Verification items for the finished model (mm, model axes). Face numbers are marked on the shaded views. Round coordinates to 2 decimals unless told otherwise and drop trailing zeros. Order: outer loops, then holes, each group sorted by start corner. A loop starts at its lowest first (then second) coordinate and runs counter-clockwise, first axis right, second up. Notation, with made-up numbers: M 55,34.5 L 72,34.5 A15 cw 72,40.5 Z; hole C 66.25,-29 d5. An arc over 180 degrees is marked long. Answer as a JSON object with one key per item and string values. Group by question number.
```python
from build123d import *

# Parameters (mm, degrees)
BOSS_EXTRUDE1_DEPTH     = 52
SHELL1_START            = 3
SHELL1_DEPTH            = 46
SKETCH2_R               = 4.5
BOSS_EXTRUDE2_DEPTH     = 52
SKETCH3_R               = 3.25
CUT_EXTRUDE1_DEPTH      = 49
SKETCH4_R               = 1.7
CUT_EXTRUDE2_DEPTH      = 91.166512631
CUT_EXTRUDE3_DEPTH      = 20
CUT_EXTRUDE3_DEPTH_BACK = 20
CUT_EXTRUDE4_DEPTH      = 3.5
SKETCH7_R               = 4
CUT_EXTRUDE5_DEPTH      = 3.5
SKETCH8_W               = 6
SKETCH8_H               = 20
BOSS_EXTRUDE3_DEPTH     = 8
SKETCH9_W               = 1.9
SKETCH9_H               = 16.6
CUT_EXTRUDE6_DEPTH      = 6
SKETCH10_R              = 5
CUT_EXTRUDE7_DEPTH      = 3.5


# Read off the part's stored shape, not the designer's step: Shell1
with BuildPart() as part:
    # Sketch1 → Boss-Extrude1 (new body)
    with BuildSketch(Plane.XY):
        with BuildLine():
            Line((-45, -55), (45, -55))
            ThreePointArc((45, -55), (52.071067812, -52.071067812), (55, -45))
            Line((55, -45), (55, -10))
            ThreePointArc((55, -10), (52.071067812, -2.928932188), (45, 0))
            Line((45, 0), (-45, 0))
            ThreePointArc((-45, 0), (-52.071067812, -2.928932188), (-55, -10))
            Line((-55, -10), (-55, -45))
            ThreePointArc((-55, -45), (-52.071067812, -52.071067812), (-45, -55))
        make_face()
    extrude(amount=BOSS_EXTRUDE1_DEPTH)

    # Shell1 outline → Shell1 (cut)
    with BuildSketch(Plane.XY.offset(SHELL1_START)):
        with BuildLine():
            Line((45, -3), (45, 0))
            Line((45, 0), (-45, 0))
            Line((-45, 0), (-45, -3))
            ThreePointArc((-45, -3), (-49.949747468, -5.050252532), (-52, -10))
            Line((-52, -10), (-52, -45))
            ThreePointArc((-52, -45), (-49.949747468, -49.949747468), (-45, -52))
            Line((-45, -52), (45, -52))
            ThreePointArc((45, -52), (49.949747468, -49.949747468), (52, -45))
            Line((52, -45), (52, -10))
            ThreePointArc((52, -10), (49.949747468, -5.050252532), (45, -3))
        make_face()
    extrude(amount=SHELL1_DEPTH, mode=Mode.SUBTRACT)

    # Sketch2 → Boss-Extrude2 (add)
    with BuildSketch(Plane(origin=(0, 0, 0), x_dir=(1, 0, 0), z_dir=(0, 1, 0))):
        with Locations(Location((-40, -8, 0), (0, 0, 270))):
            Circle(SKETCH2_R)
        with Locations(Location((40, -8, 0), (0, 0, 270))):
            Circle(SKETCH2_R)
        with Locations(Location((-40, -40, 0), (0, 0, 270))):
            Circle(SKETCH2_R)
        with Locations(Location((40, -40, 0), (0, 0, 270))):
            Circle(SKETCH2_R)
    extrude(amount=-BOSS_EXTRUDE2_DEPTH)

    # Sketch3 → Cut-Extrude1 (cut)
    with BuildSketch(Plane.XZ.offset(55)):
        with Locations(Location((-40, 8, 0), (0, 0, 270))):
            Circle(SKETCH3_R)
        with Locations(Location((40, 8, 0), (0, 0, 270))):
            Circle(SKETCH3_R)
        with Locations(Location((-40, 40, 0), (0, 0, 270))):
            Circle(SKETCH3_R)
        with Locations(Location((40, 40, 0), (0, 0, 270))):
            Circle(SKETCH3_R)
    extrude(amount=-CUT_EXTRUDE1_DEPTH, mode=Mode.SUBTRACT)

    # Sketch4 → Cut-Extrude2 (cut, through all)
    with BuildSketch(Plane.XZ.offset(6)):
        with Locations(Location((-40, 8, 0), (0, 0, 270))):
            Circle(SKETCH4_R)
        with Locations(Location((40, 8, 0), (0, 0, 270))):
            Circle(SKETCH4_R)
        with Locations(Location((-40, 40, 0), (0, 0, 270))):
            Circle(SKETCH4_R)
        with Locations(Location((40, 40, 0), (0, 0, 270))):
            Circle(SKETCH4_R)
    extrude(amount=-CUT_EXTRUDE2_DEPTH, mode=Mode.SUBTRACT)

    # Sketch5 → Cut-Extrude3 (cut, two sides: drawn at the far end of the back side and taken through both)
    with BuildSketch(Plane.XY.offset(26).offset(-CUT_EXTRUDE3_DEPTH_BACK)):
        Polygon((-51, -14), (-51, -11.5), (-55.5, -16), (-55.5, -18.5), align=None)
        Polygon((51, -14), (51, -11.5), (55.5, -16), (55.5, -18.5), align=None)
        Polygon((-51, -20), (-51, -17.5), (-55.5, -22), (-55.5, -24.5), align=None)
        Polygon((51, -20), (51, -17.5), (55.5, -22), (55.5, -24.5), align=None)
        Polygon((-51, -26), (-51, -23.5), (-55.5, -28), (-55.5, -30.5), align=None)
        Polygon((51, -26), (51, -23.5), (55.5, -28), (55.5, -30.5), align=None)
        Polygon((-51, -32), (-51, -29.5), (-55.5, -34), (-55.5, -36.5), align=None)
        Polygon((51, -32), (51, -29.5), (55.5, -34), (55.5, -36.5), align=None)
        Polygon((-51, -38), (-51, -35.5), (-55.5, -40), (-55.5, -42.5), align=None)
        Polygon((51, -38), (51, -35.5), (55.5, -40), (55.5, -42.5), align=None)
    extrude(amount=CUT_EXTRUDE3_DEPTH + CUT_EXTRUDE3_DEPTH_BACK, mode=Mode.SUBTRACT)

    # Sketch6 → Cut-Extrude4 (cut)
    with BuildSketch(Plane.XZ.offset(55)):
        with BuildLine():
            Line((-34.5, 12), (-34.5, 40))
            ThreePointArc((-34.5, 40), (-33, 41.5), (-31.5, 40))
            Line((-31.5, 40), (-31.5, 12))
            ThreePointArc((-31.5, 12), (-33, 10.5), (-34.5, 12))
        make_face()
        with BuildLine():
            Line((-28.5, 12), (-28.5, 40))
            ThreePointArc((-28.5, 40), (-27, 41.5), (-25.5, 40))
            Line((-25.5, 40), (-25.5, 12))
            ThreePointArc((-25.5, 12), (-27, 10.5), (-28.5, 12))
        make_face()
        with BuildLine():
            Line((-22.5, 12), (-22.5, 40))
            ThreePointArc((-22.5, 40), (-21, 41.5), (-19.5, 40))
            Line((-19.5, 40), (-19.5, 12))
            ThreePointArc((-19.5, 12), (-21, 10.5), (-22.5, 12))
        make_face()
        with BuildLine():
            Line((-16.5, 12), (-16.5, 40))
            ThreePointArc((-16.5, 40), (-15, 41.5), (-13.5, 40))
            Line((-13.5, 40), (-13.5, 12))
            ThreePointArc((-13.5, 12), (-15, 10.5), (-16.5, 12))
        make_face()
        with BuildLine():
            Line((-10.5, 12), (-10.5, 40))
            ThreePointArc((-10.5, 40), (-9, 41.5), (-7.5, 40))
            Line((-7.5, 40), (-7.5, 12))
            ThreePointArc((-7.5, 12), (-9, 10.5), (-10.5, 12))
        make_face()
        with BuildLine():
            Line((-4.5, 12), (-4.5, 40))
            ThreePointArc((-4.5, 40), (-3, 41.5), (-1.5, 40))
            Line((-1.5, 40), (-1.5, 12))
            ThreePointArc((-1.5, 12), (-3, 10.5), (-4.5, 12))
        make_face()
        with BuildLine():
            Line((1.5, 12), (1.5, 40))
            ThreePointArc((1.5, 40), (3, 41.5), (4.5, 40))
            Line((4.5, 40), (4.5, 12))
            ThreePointArc((4.5, 12), (3, 10.5), (1.5, 12))
        make_face()
        with BuildLine():
            Line((7.5, 12), (7.5, 40))
            ThreePointArc((7.5, 40), (9, 41.5), (10.5, 40))
            Line((10.5, 40), (10.5, 12))
            ThreePointArc((10.5, 12), (9, 10.5), (7.5, 12))
        make_face()
        with BuildLine():
            Line((31.5, 12), (31.5, 40))
            ThreePointArc((31.5, 40), (33, 41.5), (34.5, 40))
            Line((34.5, 40), (34.5, 12))
            ThreePointArc((34.5, 12), (33, 10.5), (31.5, 12))
        make_face()
    extrude(amount=-CUT_EXTRUDE4_DEPTH, mode=Mode.SUBTRACT)

    # Sketch7 → Cut-Extrude5 (cut)
    with BuildSketch(Plane(origin=(0, 0, 0), x_dir=(-1, 0, 0), z_dir=(0, 0, -1))):
        with Locations((30, -12)):
            Circle(SKETCH7_R)
        with Locations((-30, -12)):
            Circle(SKETCH7_R)
    extrude(amount=-CUT_EXTRUDE5_DEPTH, mode=Mode.SUBTRACT)

    # Sketch8 → Boss-Extrude3 (add)
    with BuildSketch(Plane(origin=(0, -52, 0), x_dir=(1, 0, 0), z_dir=(0, 1, 0))):
        with Locations((-44, -26)):
            Rectangle(SKETCH8_W, SKETCH8_H)
    extrude(amount=BOSS_EXTRUDE3_DEPTH)

    # Sketch9 → Cut-Extrude6 (cut)
    with BuildSketch(Plane(origin=(0, -44, 0), x_dir=(1, 0, 0), z_dir=(0, 1, 0))):
        with Locations((-44, -26)):
            Rectangle(SKETCH9_W, SKETCH9_H)
    extrude(amount=-CUT_EXTRUDE6_DEPTH, mode=Mode.SUBTRACT)

    # Sketch10 → Cut-Extrude7 (cut)
    with BuildSketch(Plane.XZ.offset(55)):
        with Locations(Location((20, 26, 0), (0, 0, 270))):
            Circle(SKETCH10_R)
    extrude(amount=-CUT_EXTRUDE7_DEPTH, mode=Mode.SUBTRACT)


solid = part.part
```
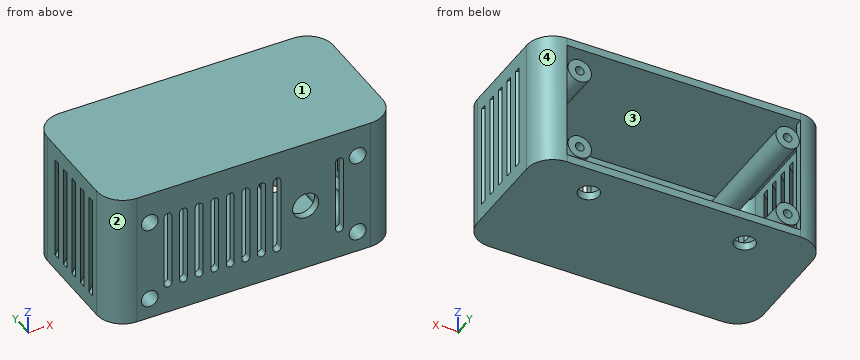
Q1. Release check for a two-part mould opening along X. For the marked faces 1, 2, 3 and 4 record: released by +X, released by -X, zero draft, split by the parting line, or undercut.
Q2. Cross-section at C-C, the plane z = 28. Give the number of separate pieces and of enclosed holes in the cut face, then the cut area to 3 significant figures.
Q3. Gauge pin test, flat ends, axial feed: pin 1 Ø3.5 at (y, z) = (-54, 29.5) entering from -X; pin 2 Ø2.5 at (y, z) = (-1, 27.5) entering from -X; pin 3 Ø6 at (x, z) = (-1, 12.5) entering from +Y. Record the tip position at first contact, or that the pin passes through.
Q4. Cross-section at B-B, the plane x = 20. Record the cut outline in (y, z), then the cut area to 3 significant figures.
Q5. Thickness scan on line 1 (Z direction, x = -4, y = -47.5); line 2 (X direction, y = -12, z = 47.5); line 3 (Z direction, x = -38.5, y = -38). Record the ranges inside material, lowest first. Write a range as from..to.
Q6. Cross-section at A-A, the plane x = -21. Record the cut outline in (y, z).
Conclusion:
{
 "1": {"face 1": "zero draft", "face 2": "released by -X", "face 3": "undercut", "face 4": "released by +X"},
 "2": {"separate pieces": "21", "enclosed holes": "0", "area": "493 mm2"},
 "3": {"pin 1": "x = -51.89", "pin 2": "x = -51.32", "pin 3": "y = -52"},
 "4": {"outline": "M -55,0 L 0,0 L 0,3 L -52,3 L -52,21 L -55,21 Z; M -55,31 L -52,31 L -52,49 L 0,49 L 0,52 L -55,52 Z", "area": "438 mm2"},
 "5": {"line 1": "0..3, 49..52", "line 2": "-55..-52, 52..55", "line 3": "0..3, 3.76..5.12, 10.88..12.24, 35.76..37.12, 42.88..44.24, 49..52"},
 "6": {"outline": "M -55,0 L 0,0 L 0,3 L -52,3 L -52,10.5 L -55,10.5 Z; M -55,41.5 L -52,41.5 L -52,49 L 0,49 L 0,52 L -55,52 Z"}
}
